Input: part model. Units: mm. Frame: model coordinates. A direction names the side the tool comes from. Coordinates: 2 decimals unless noted, no trailing zeros. Order: outer loops, then holes, each group sorted by start corner. A loop starts at its lowest first (then second) coordinate and runs counter-clockwise, first axis right, second up. Notation, with made-up numbers: (88, 53) -> (131, 53) arc R31 cw to (131, 91) -> close; hole circle Ø1 at (-37.75, 22). An arc over 180 degrees is marked (long way). One line per item, written item: value. Start each with the question number.
Autodesk Inventor part; units mm, degrees
ref_plane "Work Plane1" through (0, 0, 17.5) normal (0, 0, -1) x (-1, 0, 0)
ref_plane "YZ Plane" through (0, 0, 0) normal (1, 0, 0) x (0, 1, 0)
ref_plane "XZ Plane" through (0, 0, 0) normal (0, 1, 0) x (-1, 0, 0)
sketch "Sketch1" plane through (0, 0, 0) normal (0, 0, 1) x (1, 0, 0)
  line L0 (0, 0) -> (0, 20)
  arc A0 (10.3297, 33.6293) -> (0, 20) centre (26.5688, 10.5925) ccw
  line L1 (10.3297, 33.6293) -> (13.2894, 33.6293)
  arc A1 (12.1727, 30.4088) -> (10.3814, 12.1465) centre (23.0461, 20.1232) ccw
  line L2 (10.3814, 12.1465) -> (19.3334, 0)
  line L3 (19.3334, 0) -> (0, 0)
  line L4 (12.1727, 30.4088) -> (14.8574, 30.4088)
  line L5 (14.8574, 30.4088) -> (16.1699, 33.6293)
  line L6 (16.1699, 33.6293) -> (13.2894, 33.6293)
  circle A2 centre (7, 5) radius 3.5
  dimension "d0" = 20
  dimension "d1" = 7
  dimension "d2" = 14.9674
  dimension "d3" = 28.1852
  dimension "d4" = 67.827
  dimension "d5" = 10.2856
  dimension "d6" = 7
  dimension "d7" = 5
  dimension "d8" = 53.61
  dimension "d9" = 3.2206
extrude "Extrusion1" add sketch "Sketch1" along normal blind 35
ref_plane "Work Plane1" through (0, 0, 17.5) normal (0, 0, -1) x (-1, 0, 0)
sketch "Sketch2" plane through (0, 0, 17.5) normal (0, 0, -1) x (-1, 0, 0)
  line L0 (-1, 0) -> (-21, 0)
  line L1 (-21, 0) -> (-21, 14)
  line L2 (-21, 14) -> (-1, 14)
  line L3 (-1, 14) -> (-1, 0)
  line L4 (0, 0) -> (-25.0349, 0) construction
  dimension "d12" = 20
  dimension "d13" = 14
  dimension "d15" = 1
extrude "Extrusion2" cut sketch "Sketch2" along normal mid plane 25
1) Mould query, pull axis Y, two halves, no side actions, for faces 1 (the flat face through (1, 7, 18)), 2 (the cylindrical face through (3.503, 4.846, 32.465)), 3 (the cylindrical face through (4.033, 27.52, 17.255)). Classes: +Y half, -Y half, draft (parallel to the pull), parting line (faces both ways), or undercut.
2) Access query for faces 4 (the flat face through (13, 30.409, 17)), 5 (the flat face through (0.4, 0, 18.7)), 6 (the flat face through (5, 14, 18)). Directions: +Z, -Z, +X, -X, +Y, -Y. A direction counts if a zero-diameter tool reaches every point of the face in a straight line with its end or side. Return the directions, or none.
3) Section query D-D, the plane z = 11.5. Return the cut outline in (x, y), plus the area to 3 significant figures.
4) Section query C-C, the plane y = 3.5. Return the cut outline in (x, z).
5) Ray query, line 1 along Z through (x, y) = (2.5, 8); line 2 along X through (y, z) = (9, 14.5); line 3 along Y through (x, z) = (13.5, 6). Return the intervals inside material, ascending. Write a range as from..to.
6) Section query B-B, the plane x = 7. Return the cut outline in (y, z), plus the area to 3 significant figures.
7) Section query A-A, the plane z = 4.5. Return the cut outline in (x, y).
8) Pin query (flat end, axial travel): pin 1 Ø7 at (y, z) = (4.5, 13.5) entering from +X; pin 2 Ø8 at (y, z) = (24, 18.5) entering from +X; pin 3 Ø1.3 at (x, z) = (13.5, 19) entering from -Y; pin 4 Ø4 at (x, y) = (11, 19) entering from -Z. Return the tip coordinate at first contact, or that it passes through.
Entries:
1. face 1: draft
1. face 2: undercut
1. face 3: +Y half
2. face 4: +Z, -Z, +X
2. face 5: +Z, -Z, +X, -X, -Y
2. face 6: +X, -Y
3. outline: (0, 0) -> (1, 0) -> (1, 14) -> (9.39, 14) arc R14.97 cw to (12.17, 30.41) -> (14.86, 30.41) -> (16.17, 33.63) -> (10.33, 33.63) arc R28.19 ccw to (0, 20) -> close
3. area: 157 mm2
4. outline: (0, 0) -> (3.84, 0) -> (3.84, 5) -> (1, 5) -> (1, 30) -> (3.84, 30) -> (3.84, 35) -> (0, 35) -> close; (10.16, 0) -> (16.75, 0) -> (16.75, 5) -> (10.16, 5) -> close; (10.16, 30) -> (16.75, 30) -> (16.75, 35) -> (10.16, 35) -> close
5. line 1: z = 0..5, 30..35
5. line 2: x = 0..1
5. line 3: y = 30.41..33.63
6. outline: (0, 0) -> (1.5, 0) -> (1.5, 5) -> (0, 5) -> close; (0, 30) -> (1.5, 30) -> (1.5, 35) -> (0, 35) -> close; (8.5, 0) -> (30.88, 0) -> (30.88, 35) -> (8.5, 35) -> (8.5, 30) -> (14, 30) -> (14, 5) -> (8.5, 5) -> close
6. area: 661 mm2
7. outline: (0, 0) -> (19.33, 0) -> (10.38, 12.15) arc R14.97 cw to (12.17, 30.41) -> (14.86, 30.41) -> (16.17, 33.63) -> (10.33, 33.63) arc R28.19 ccw to (0, 20) -> close; hole circle Ø7 at (7, 5)
8. pin 1: stops at x = 1
8. pin 2: stops at x = 10.32
8. pin 3: stops at y = 30.41
8. pin 4: passes through
